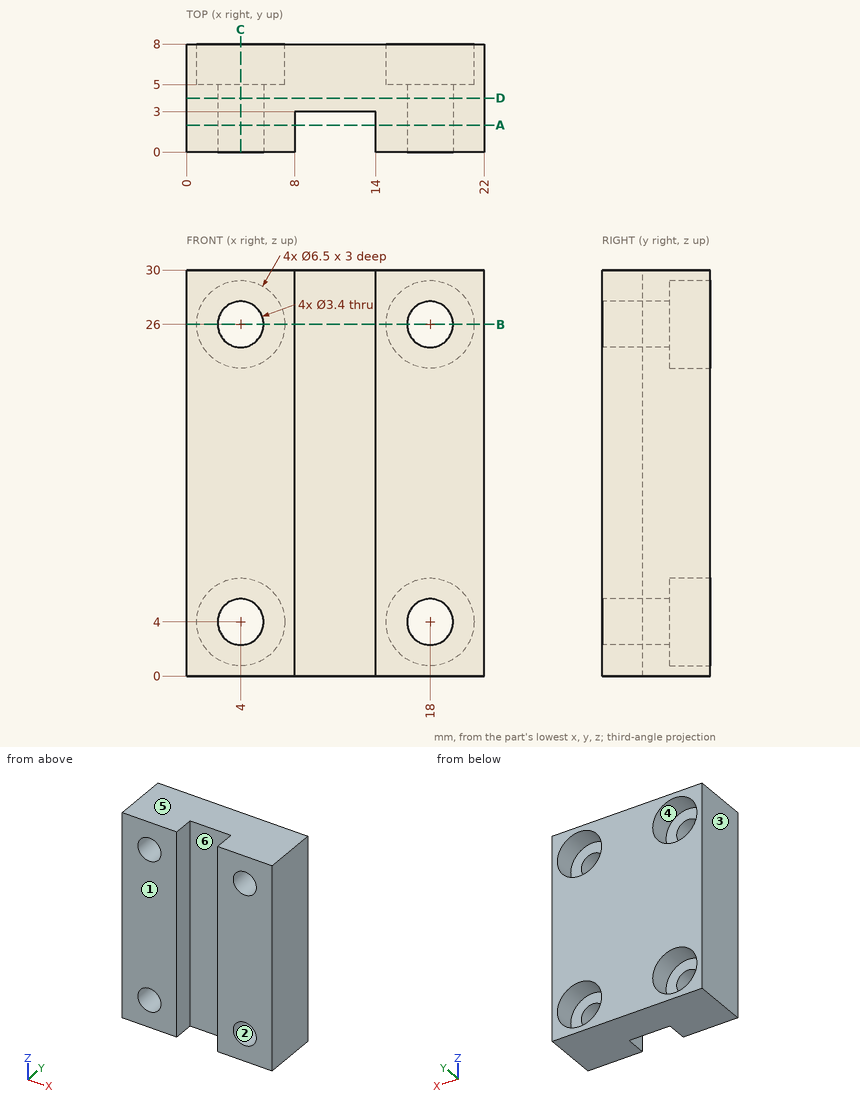
Design review of the part shown in the three views and the two pictorial views. Dimensions are in mm from the part's minimum x, y and z. A direction names the side the tool comes from. Give positions to 0.01 mm unless a question says otherwise; leave off trailing zeros. Loops run counter-clockwise (first coordinate to the right, second up) from the corner with the lowest first, then second, coordinate; pieces in that order, holes last. Notation, with made-up numbers: M 12.25,-21 L 18.25,-21 A30 ccw 18.25,6 Z; hole C 4.5,9.25 d9. An arc over 180 degrees is marked long. Put each result on its own line as item: value. Start each with the question number.
(1) Wall thickness on L1, parallel to Z at x = 4, y = 6.65; L2, parallel to Z at x = 4, y = 2.5; L3, parallel to X at y = 5.75, z = 26: over which ranges is each line inside the solid? List them lowest first.
(2) For pin 1 (1.8 mm diameter, centred on x = 11.5, z = 10.5, fed in from -Y); pin 2 (3 mm diameter, centred on x = 19, z = 5.5, fed in from +Y); pin 3 (2 mm diameter, centred on x = 3, z = 2.5, fed in from +Y); pin 4 (3 mm diameter, centred on x = 18, z = 4, fed in from -Y), all flat-tipped, find the tip position at first contact; note any pin that passes through.
(3) Add section D-D, the plane y = 4. Write out the cut boundary in (x, z).
(4) Add section B-B, the plane z = 26. Write out the cut boundary in (x, y), then the cut area to 3 significant figures.
(5) Machinability: for the marked faces 4, 5 and 6, which of the approach directions +Z, -Z, +X, -X, +Y, -Y give a long, thin tool a straight path to every point of the face, cutting with its end or side? Answer none if there is none.
(6) Add section C-C, the plane x = 4. Write out the cut boundary in (y, z).
(7) The part is to be moulded in two halves that separate along X. For the marked faces 1, 2 and 3, say which applies: +X half, -X half, draft (parallel to the pull), parting line (faces both ways), or undercut.
(8) Add section A-A, the plane y = 2. Write out the cut boundary in (x, z).
Result:
1. L1: z = 0 to 0.75, 7.25 to 22.75, 29.25 to 30
1. L2: z = 0 to 2.3, 5.7 to 24.3, 27.7 to 30
1. L3: x = 0 to 0.75, 7.25 to 14.75, 21.25 to 22
2. pin 1: stops at y = 3
2. pin 2: stops at y = 8
2. pin 3: stops at y = 5
2. pin 4: passes through
3. outline: M 0,0 L 22,0 L 22,30 L 0,30 Z; hole C 4,4 d3.4; hole C 4,26 d3.4; hole C 18,4 d3.4; hole C 18,26 d3.4
4. outline: M 0,0 L 2.3,0 L 2.3,5 L 0.75,5 L 0.75,8 L 0,8 Z; M 5.7,0 L 8,0 L 8,3 L 14,3 L 14,0 L 16.3,0 L 16.3,5 L 14.75,5 L 14.75,8 L 7.25,8 L 7.25,5 L 5.7,5 Z; M 19.7,0 L 22,0 L 22,8 L 21.25,8 L 21.25,5 L 19.7,5 Z
4. area: 85.0 mm^2
5. face 4: +Y
5. face 5: +Z, +X, -X, +Y, -Y
5. face 6: +Z, -Z, -Y
6. outline: M 0,0 L 8,0 L 8,0.75 L 5,0.75 L 5,2.3 L 0,2.3 Z; M 0,5.7 L 5,5.7 L 5,7.25 L 8,7.25 L 8,22.75 L 5,22.75 L 5,24.3 L 0,24.3 Z; M 0,27.7 L 5,27.7 L 5,29.25 L 8,29.25 L 8,30 L 0,30 Z
7. face 1: draft
7. face 2: undercut
7. face 3: -X half
8. outline: M 0,0 L 8,0 L 8,30 L 0,30 Z; M 14,0 L 22,0 L 22,30 L 14,30 Z; hole C 4,4 d3.4; hole C 4,26 d3.4; hole C 18,4 d3.4; hole C 18,26 d3.4
